Part model, mm, in its own coordinate system. A direction names the side the tool comes from. Round coordinates to 2 decimals unless told otherwise and drop trailing zeros. Order: outer loops, then holes, each group sorted by start corner. A loop starts at its lowest first (then second) coordinate and runs counter-clockwise, first axis right, second up. Notation, with made-up numbers: (63, 35.5) - (87, 35.5) arc R13 ccw to (87, 49.5) - close; hole circle Ø5 at (-37, -5.5). An arc over 180 degrees is marked (long way). Return JSON: item names as keys, results as strings. Group by question number.
Item 1: Drop flat-ended pins along their axis: pin 1 (4.5 mm diameter, centred on x = -67.94, y = 54.41, fed in from +Z); pin 2 (2.5 mm diameter, centred on x = -66.61, y = -50.27, fed in from -Z). Give the stop position or say it passes through.
Item 2: Saw through at C-C on x = 61. List the corners of the cut face in (y, z), and give its area (3 significant figures).
Item 3: Probe probe 1 along X at (y, z) = (143.5, 1.55); probe 2 along Y at (x, z) = (4, 1.7); probe 3 along Y at (x, z) = (-15, 1.7). List the from-to ranges inside material, lowest first.
Item 4: Saw through at A-A on y = -58.5. List the corners of the cut face in (x, z).
Item 5: Two-plate mould, pull along X, no slides. Class faces 3 (the face through (20.65, 73.59, 0.99)), 4 (the face through (-58, 19, 2)), 5 (the face through (-45.318, 163.147, 0.986)): released by +X, released by -X, zero draft, split by the parting line, or undercut.
Item 6: Tool access for faces 1 (the face through (-58, 19, 0)), 2 (the face through (10.44, 42.98, 0.99)): list every direction of +Z, -Z, +X, -X, +Y, -Y with a clear straight run to the whole face (end or side of a thin tool).
Item 7: Saw through at B-B on z = 1.6. State how many separate pieces and enclosed holes the cut face has, and give its area (3 significant figures).
```python
from build123d import *

# Parameters (mm, degrees)
SKETCH1_R           = 120.00268075
SKETCH1_R_2         = 1.475
BOSS_EXTRUDE1_DEPTH = 2


with BuildPart() as part:
    # Sketch1 → Boss-Extrude1 (new body)
    with BuildSketch(Plane.XY):
        with Locations((-29.695990648, 44.165693097)):
            Circle(SKETCH1_R)
        with Locations((-131.117764712, 78.090450262)):
            Circle(SKETCH1_R_2, mode=Mode.SUBTRACT)
        with Locations((-93.581586999, 46.593857387)):
            Circle(SKETCH1_R_2, mode=Mode.SUBTRACT)
        with Locations((-56.299905637, 91.024435088)):
            Circle(SKETCH1_R_2, mode=Mode.SUBTRACT)
        with Locations((-93.83608335, 122.521027963)):
            Circle(SKETCH1_R_2, mode=Mode.SUBTRACT)
        with Locations((-110.045426455, -36.150986818)):
            Circle(SKETCH1_R_2, mode=Mode.SUBTRACT)
        with Locations((-122.090933715, -9.178552154)):
            Circle(SKETCH1_R_2, mode=Mode.SUBTRACT)
        with Locations((-90.443310675, -16.556862192)):
            Circle(SKETCH1_R_2, mode=Mode.SUBTRACT)
        with Locations((-86.537268392, -54.200307389)):
            Circle(SKETCH1_R_2, mode=Mode.SUBTRACT)
        with Locations((-66.607427563, -50.274288778)):
            Circle(SKETCH1_R_2, mode=Mode.SUBTRACT)
        with Locations((-74.107508579, -7.739215663)):
            Circle(SKETCH1_R_2, mode=Mode.SUBTRACT)
        with Locations((-139.426993706, 14.739380466)):
            Circle(SKETCH1_R_2, mode=Mode.SUBTRACT)
        with Locations((-112.656926125, 21.918248387)):
            Circle(SKETCH1_R_2, mode=Mode.SUBTRACT)
        with Locations((-143.304084809, 44.12270283)):
            Circle(SKETCH1_R_2, mode=Mode.SUBTRACT)
        with BuildLine():
            ThreePointArc((-66.409488535, 24.672278037), (-65.290263608, 24.819626794), (-64.394660767, 24.132406564))
            ThreePointArc((-64.394660767, 24.132406564), (-64.247310389, 23.013187685), (-64.934521394, 22.117585057))
            Line((-64.934521394, 22.117585057), (-69.391907416, 19.544061572))
            Line((-69.391907416, 19.544061572), (-74.290393291, 16.715919433))
            ThreePointArc((-74.290393291, 16.715919433), (-75.409651382, 16.56856631), (-76.305280761, 17.255806904))
            ThreePointArc((-76.305280761, 17.255806904), (-76.452633885, 18.375064995), (-75.765393291, 19.270694374))
            Line((-75.765393291, 19.270694374), (-70.866896569, 22.098842775))
            Line((-70.866896569, 22.098842775), (-66.409488535, 24.672278037))
        make_face(mode=Mode.SUBTRACT)
        with Locations((-39.944701954, 5.916981791)):
            Circle(SKETCH1_R_2, mode=Mode.SUBTRACT)
        with Locations((27.145287096, -54.200307389)):
            Circle(SKETCH1_R_2, mode=Mode.SUBTRACT)
        with Locations((50.653445159, -36.150986818)):
            Circle(SKETCH1_R_2, mode=Mode.SUBTRACT)
        with Locations((31.051329379, -16.556862192)):
            Circle(SKETCH1_R_2, mode=Mode.SUBTRACT)
        with Locations((35.640132692, -22.598732381)):
            Circle(SKETCH1_R_2, mode=Mode.SUBTRACT)
        with BuildLine():
            ThreePointArc((-23.271008074, 7.727806236), (-45.332866332, 10.632304977), (-61.738930588, 25.665693097))
            ThreePointArc((-61.738930588, 25.665693097), (-66.555194477, 47.390455579), (-58.039635043, 67.948834656))
            ThreePointArc((-58.039635043, 67.948834656), (-42.381951879, 78.922942523), (-23.336458345, 80.615060018))
            Line((-23.336458345, 80.615060018), (1.683916538, 78.448698496))
            ThreePointArc((1.683916538, 78.448698496), (20.808272191, 73.324342843), (15.683916538, 54.19998719))
            Line((15.683916538, 54.19998719), (5.049853209, 31.448526168))
            ThreePointArc((5.049853209, 31.448526168), (-5.938310295, 15.800703687), (-23.271008074, 7.727806236))
        make_face(mode=Mode.SUBTRACT)
        with Locations((16.677076311, 47.845185022)):
            Circle(SKETCH1_R_2, mode=Mode.SUBTRACT)
        with Locations((30.83159843, 4.671820563)):
            Circle(SKETCH1_R_2, mode=Mode.SUBTRACT)
        with Locations((53.264944829, 21.918248387)):
            Circle(SKETCH1_R_2, mode=Mode.SUBTRACT)
        with Locations((80.03501241, 14.739380466)):
            Circle(SKETCH1_R_2, mode=Mode.SUBTRACT)
        with Locations((83.912103514, 44.12270283)):
            Circle(SKETCH1_R_2, mode=Mode.SUBTRACT)
        with Locations((-67.944701954, 54.414404403)):
            Circle(SKETCH1_R_2, mode=Mode.SUBTRACT)
        with Locations((-51.909606098, 127.135693097)):
            Circle(SKETCH1_R_2, mode=Mode.SUBTRACT)
        with Locations((-86.462807065, 142.57468385)):
            Circle(SKETCH1_R_2, mode=Mode.SUBTRACT)
        with Locations((-59.077557898, 153.908685644)):
            Circle(SKETCH1_R_2, mode=Mode.SUBTRACT)
        with Locations((-3.322923689, 82.486201173)):
            Circle(SKETCH1_R_2, mode=Mode.SUBTRACT)
        with Locations((-7.482375198, 127.135693097)):
            Circle(SKETCH1_R_2, mode=Mode.SUBTRACT)
        with Locations((-0.314423397, 153.908685644)):
            Circle(SKETCH1_R_2, mode=Mode.SUBTRACT)
        with Locations((27.070825769, 142.57468385)):
            Circle(SKETCH1_R_2, mode=Mode.SUBTRACT)
    extrude(amount=BOSS_EXTRUDE1_DEPTH)


solid = part.part
```
Filled in:
{
 "1": {"pin 1": "stops at z = 2", "pin 2": "passes through"},
 "2": {"outline": "(-34.41, 0) - (122.75, 0) - (122.75, 2) - (-34.41, 2) - close", "area": "314 mm^2"},
 "3": {"probe 1": "x = -97.03 to -87.61, -85.31 to 25.92, 28.22 to 37.63", "probe 2": "y = -71.01 to 28.88, 79.52 to 159.34", "probe 3": "y = -74.93 to 10.21, 79.89 to 163.27"},
 "4": {"outline": "(-91.83, 0) - (32.44, 0) - (32.44, 2) - (-91.83, 2) - close"},
 "5": {"face 3": "undercut", "face 4": "zero draft", "face 5": "split by the parting line"},
 "6": {"face 1": "-Z, +X, -X, +Y, -Y", "face 2": "+Z, -Z"},
 "7": {"separate pieces": "1", "enclosed holes": "33", "area": "40,000 mm^2"}
}
